CAD build for the part. Positions are in the model's coordinates, mm. Give positions to 0.01 mm unless a question says otherwise; leave off trailing zeros. Loops run counter-clockwise (first coordinate to the right, second up) from the corner with the lowest first, then second, coordinate; pieces in that order, holes last. Notation, with made-up numbers: M 73.5,21.5 L 98.5,21.5 A17 ccw 98.5,29.5 Z; hole C 17,18.25 d1. An arc over 180 degrees is marked long. Answer as CSV lines item,"result".
```python
from build123d import *

# Parameters (mm, degrees)
F1_DEPTH = 1.27
F2_R     = 0.508


with BuildPart() as f1:
    # F0 (on Front) → F1 (new body)
    with BuildSketch(Plane.XZ):
        Polygon((-8.3281235051, 34.2946868681), (-8.3281235051, 35.56), (-8.3281235051, 38.1), (-9.5981235051, 38.1), (-9.5981235051, 35.56), (-43.8881235051, 35.56), (-43.8881235051, 34.2946868681), (-9.5981235051, 34.2946868681), (-9.5981235051, 8.8946868681), (-43.8881235051, 8.8946868681), (-43.8881235051, 7.6246868681), (-9.5981235051, 7.6246868681), (-9.5981235051, 7.1166868681), (-10.4112418222, 6.35), (-9.5981235051, 6.35), (-9.5981235051, 0), (-8.3281235051, 0), (-8.3281235051, 6.35), (-7.5661235051, 6.35), (-8.3281235051, 7.1166868681), (-8.3281235051, 7.6246868681), (-8.3281235051, 8.8946868681), align=None)
        Polygon((27.2318764949, 34.2946868681), (27.2318764949, 35.56), (27.2318764949, 38.1), (25.9618764949, 38.1), (25.9618764949, 35.56), (-8.3281235051, 35.56), (-8.3281235051, 34.2946868681), (25.9618764949, 34.2946868681), (25.9618764949, 8.8946868681), (-8.3281235051, 8.8946868681), (-8.3281235051, 7.6246868681), (25.9618764949, 7.6246868681), (25.9618764949, 7.1166868681), (25.1487581778, 6.35), (25.9618764949, 6.35), (25.9618764949, 0), (27.2318764949, 0), (27.2318764949, 6.35), (27.9938764949, 6.35), (27.2318764949, 7.1166868681), (27.2318764949, 7.6246868681), (27.2318764949, 8.8946868681), align=None)
        Polygon((62.7918764949, 34.2946868681), (62.7918764949, 35.56), (62.7918764949, 38.1), (61.5218764949, 38.1), (61.5218764949, 35.56), (27.2318764949, 35.56), (27.2318764949, 34.2946868681), (61.5218764949, 34.2946868681), (61.5218764949, 8.8946868681), (27.2318764949, 8.8946868681), (27.2318764949, 7.6246868681), (61.5218764949, 7.6246868681), (61.5218764949, 7.1166868681), (60.7087581778, 6.35), (61.5218764949, 6.35), (61.5218764949, 0), (62.7918764949, 0), (62.7918764949, 6.35), (63.5538764949, 6.35), (62.7918764949, 7.1166868681), (62.7918764949, 7.6246868681), (62.7918764949, 8.8946868681), align=None)
        Polygon((98.3518764949, 7.1166868681), (98.3518764949, 38.1), (97.0818764949, 38.1), (97.0818764949, 35.56), (62.7918764949, 35.56), (62.7918764949, 34.2946868681), (97.0818764949, 34.2946868681), (97.0818764949, 8.8946868681), (62.7918764949, 8.8946868681), (62.7918764949, 7.6246868681), (97.0818764949, 7.6246868681), (97.0818764949, 7.1166868681), (96.2687581778, 6.35), (97.0818764949, 6.35), (97.0818764949, 0), (98.3518764949, 0), (98.3518764949, 6.35), (99.1138764949, 6.35), align=None)
    extrude(amount=F1_DEPTH)

    # F2
    f2_edges = [f1.edges().sort_by_distance(p)[0] for p in [
        (-26.743124, -1.27, 34.294687),
        (-26.743124, -1.27, 35.56),
        (-9.598124, -1.27, 21.594687),
        (-8.328124, -1.27, 21.594687),
        (-26.743124, -1.27, 8.894687),
        (-26.743124, -1.27, 7.624687),
        (-9.598124, -1.27, 36.83),
        (25.961876, -1.27, 36.83),
        (61.521876, -1.27, 36.83),
        (27.231876, -1.27, 36.83),
        (-8.328124, -1.27, 36.83),
        (8.816876, -1.27, 35.56),
        (8.816876, -1.27, 34.294687),
        (8.816876, -1.27, 8.894687),
        (8.816876, -1.27, 7.624687),
        (-8.328124, -1.27, 3.175),
        (27.231876, -1.27, 3.175),
        (62.791876, -1.27, 3.175),
        (44.376876, -1.27, 7.624687),
        (44.376876, -1.27, 8.894687),
        (44.376876, -1.27, 34.294687),
        (44.376876, -1.27, 35.56),
        (62.791876, -1.27, 36.83),
        (79.936876, -1.27, 35.56),
        (79.936876, -1.27, 34.294687),
        (62.791876, -1.27, 21.594687),
        (61.521876, -1.27, 21.594687),
        (79.936876, -1.27, 8.894687),
        (79.936876, -1.27, 7.624687),
        (61.521876, -1.27, 3.175),
        (25.961876, -1.27, 3.175),
        (27.231876, -1.27, 21.594687),
        (25.961876, -1.27, 21.594687),
        (-9.598124, -1.27, 3.175),
        (97.081876, -1.27, 36.83),
        (97.081876, -1.27, 21.594687),
        (98.351876, -1.27, 3.175),
        (98.351876, -1.27, 22.608343),
        (97.081876, -1.27, 3.175),
    ]]
    fillet(f2_edges, radius=F2_R)


solid = f1.part
```
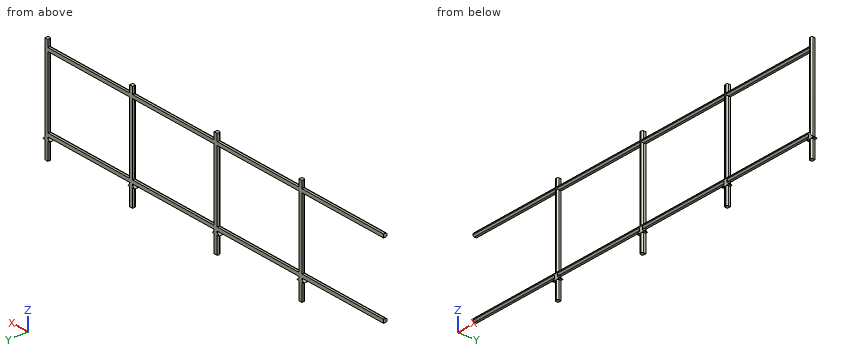
Q1. Cut at B-B (x = -31.5). Write the cut outline in (y, z), and give its area (3 significant figures).
Solution:
outline,"M -1.27,8.13 A0.51 ccw -0.76,7.62 L 0,7.62 L 0,8.89 L -0.76,8.89 A0.51 ccw -1.27,8.39 Z; M -1.27,34.8 A0.51 ccw -0.76,34.29 L 0,34.29 L 0,35.56 L -0.76,35.56 A0.51 ccw -1.27,35.05 Z"
area,"3.00 mm²"
Q2. Pin check, flat tips, straight feed: P1, Ø1.5, axis at x = 24, z = 19, coming from the -Y side; P2, Ø0.6, axis at y = -0.5, z = 37, coming from the -X side; P3, Ø0.6, axis at x = 77.5, y = -0.5, coming from the +Z side; P4, Ø0.5, axis at y = -0.5, z = 8, coming from the +X side. Stop position of each tip, or through.
Solution:
P1,"passes through"
P2,"stops at x = -9.6"
P3,"stops at z = 35.56"
P4,"stops at x = 98.35"
Q3. Cut at A-A (z = 19). Write the cut outline in (x, y).
Solution:
outline,"M -9.6,-0.76 A0.51 ccw -9.09,-1.27 L -8.84,-1.27 A0.51 ccw -8.33,-0.76 L -8.33,0 L -9.6,0 Z; M 25.96,-0.76 A0.51 ccw 26.47,-1.27 L 26.72,-1.27 A0.51 ccw 27.23,-0.76 L 27.23,0 L 25.96,0 Z; M 61.52,-0.76 A0.51 ccw 62.03,-1.27 L 62.28,-1.27 A0.51 ccw 62.79,-0.76 L 62.79,0 L 61.52,0 Z; M 97.08,-0.76 A0.51 ccw 97.59,-1.27 L 97.84,-1.27 A0.51 ccw 98.35,-0.76 L 98.35,0 L 97.08,0 Z"
Q4. Cut at C-C (y = -1). Give the number of separate pieces and of enclosed holes in the cut face, and give its area (3 significant figures).
Solution:
separate pieces,"1"
enclosed holes,"3"
area,"495 mm²"
Q5. Wall check: line 1 (X direction, y = -0.85, z = 18.5); line 2 (X direction, y = -0.25, z = 34); line 3 (Z direction, x = 50, y = -0.2). Give the ranges that are in metal, low to high. Write a range as [from, to].
Solution:
line 1,"x = [-9.59, -8.34], [25.97, 27.22], [61.53, 62.78], [97.09, 98.34]"
line 2,"x = [-9.6, -8.33], [25.96, 27.23], [61.52, 62.79], [97.08, 98.35]"
line 3,"z = [7.62, 8.89], [34.29, 35.56]"
